Here's how the part is built. I have some questions about the finished solid (model axes, mm). A direction names the side the tool comes from. Coordinates: 2 decimals unless noted, no trailing zeros. Loops run counter-clockwise (first coordinate to the right, second up) from the corner with the lowest first, then second, coordinate; pieces in that order, holes last. Notation, with made-up numbers: M -32.5,70.25 L 25.5,70.25 A23 ccw 25.5,99.25 Z; hole C -34.5,6.25 d1. An arc over 180 degrees is marked long. Use CSV: the item, a comma, the result in double quotes. Start each with the question number.
Q1. If we section it at A-A (z = -26.67): Please give me the cut outline in (x, y), and give its area (3 significant figures).
Q2. Which directions (+Z, -Z, +X, -X, +Y, -Y) give clear straight access to the entire face, cutting with the end or side of a thin tool? Please do faces 1 (the cylindrical face through (4.74, 4.25, -4.98)), 2 (the flat face through (3.175, 3, -6)).
Q3. Please list where these lines run through material, in increasing order: probe 1 along Y at (x, z) = (4.2, -3.81); probe 2 along Z at (x, y) = (4.5, 2.5); probe 3 along Z at (x, y) = (3.5, 3). Write a range as [from, to].
Q4. For pin 1 Ø3.5 at (x, y) = (1.5, 3) entering from +Z; pin 2 Ø3 at (y, z) = (4, -8.5) entering from -X (3 decimals), each with a flat end and sliding along its axis, tell me the tip position at first contact or that it passes through.
Q5. If we mould it in two halves opening along Z, with no side actions, what happens to faces 3 (the cylindrical face through (3.131, 3.245, -28.256)), 4 (the flat face through (5, 3, 0)), 5 (the flat face through (3, 3, -30.48))? For each: +Z half, -Z half, draft (parallel to the pull), parting line (faces both ways), or undercut.
Q6. If we section it at C-C (y = 1.25): Please give me the cut outline in (x, z) (3 decimals).
from build123d import *

# Parameters (mm, degrees)
SKETCH1_W                        = 30.48
SKETCH1_H                        = 6.35
BOSS_EXTRUDE1_DEPTH              = 6.35
F_1_8_0_125_DIAMETER_HOLE1_D     = 3.175
F_1_8_0_125_DIAMETER_HOLE1_DEPTH = 70.104
F_1_8_0_125_DIAMETER_HOLE1_TIP   = 0.953866233
SKETCH4_W                        = 12.7
SKETCH4_H                        = 6.35
CUT_EXTRUDE1_DEPTH               = 3.175
F_1_8_0_125_DIAMETER_HOLE2_D     = 3.175
F_1_8_0_125_DIAMETER_HOLE2_DEPTH = 70.104
F_1_8_0_125_DIAMETER_HOLE2_TIP   = 0.953866233


with BuildPart() as part:
    # Sketch1 → Boss-Extrude1 (new body)
    with BuildSketch(Plane(origin=(0, 0, 0), x_dir=(0, 0, -1), z_dir=(1, 0, 0))):
        with Locations((15.24, 3.175)):
            Rectangle(SKETCH1_W, SKETCH1_H)
    extrude(amount=BOSS_EXTRUDE1_DEPTH)

    # 1/8 (0.125) Diameter Hole1
    with Locations(Plane(origin=(6.35, 0, 0), x_dir=(0, 0, -1), z_dir=(1, 0, 0))):
        with Locations((3.81, 3.175)):
            Hole(F_1_8_0_125_DIAMETER_HOLE1_D / 2, depth=F_1_8_0_125_DIAMETER_HOLE1_DEPTH)
            with Locations((0, 0, -(F_1_8_0_125_DIAMETER_HOLE1_DEPTH + F_1_8_0_125_DIAMETER_HOLE1_TIP / 2))):  # 118° drill point
                Cone(0, F_1_8_0_125_DIAMETER_HOLE1_D / 2, F_1_8_0_125_DIAMETER_HOLE1_TIP, mode=Mode.SUBTRACT)

    # Sketch4 → Cut-Extrude1 (cut)
    with BuildSketch(Plane.ZY):
        with Locations((-6.35, 3.175)):
            Rectangle(SKETCH4_W, SKETCH4_H)
    extrude(amount=-CUT_EXTRUDE1_DEPTH, mode=Mode.SUBTRACT)

    # 1/8 (0.125) Diameter Hole2
    with Locations(Plane(origin=(6.35, 0, 0), x_dir=(0, 0, -1), z_dir=(1, 0, 0))):
        with Locations((26.67, 3.175), (33.02, 3.175)):
            Hole(F_1_8_0_125_DIAMETER_HOLE2_D / 2, depth=F_1_8_0_125_DIAMETER_HOLE2_DEPTH)
            with Locations((0, 0, -(F_1_8_0_125_DIAMETER_HOLE2_DEPTH + F_1_8_0_125_DIAMETER_HOLE2_TIP / 2))):  # 118° drill point
                Cone(0, F_1_8_0_125_DIAMETER_HOLE2_D / 2, F_1_8_0_125_DIAMETER_HOLE2_TIP, mode=Mode.SUBTRACT)


solid = part.part
Results below:
1,outline,"M 0,0 L 6.35,0 L 6.35,1.59 L 0,1.59 Z; M 0,4.76 L 6.35,4.76 L 6.35,6.35 L 0,6.35 Z"
1,area,"20.2 mm^2"
2,face 1,"+X, -X"
2,face 2,"+Z, -X, +Y, -Y"
3,probe 1,"[0, 1.59], [4.76, 6.35]"
3,probe 2,"[-30.48, -28.11], [-25.23, -5.25], [-2.37, 0]"
3,probe 3,"[-30.48, -28.25], [-25.09, -5.39], [-2.23, 0]"
4,pin 1,"z = 0"
4,pin 2,"x = 3.175"
5,face 3,"undercut"
5,face 4,"+Z half"
5,face 5,"-Z half"
6,outline,"M 0,-30.48 L 6.35,-30.48 L 6.35,0 L 3.175,0 L 3.175,-12.7 L 0,-12.7 Z"
